Check sheet for the modelled part. Datum: model origin and axes. Units: mm. A direction names the side the tool comes from. Round coordinates to 2 decimals unless told otherwise and drop trailing zeros. Write each loop counter-clockwise with the first axis right and the second up, starting at its lowest first coordinate (ties: lowest second). Pieces come first, ordered by that corner, then holes.
Item 1: Tool access check on faces 1 (the flat face through (23.855, -8, 9)), 2 (the flat face through (10, 30.184, 9)), 3 (the flat face through (-5.901, 33, 7)). Record the directions out of +Z, -Z, +X, -X, +Y, -Y that give a thin tool (end or side, any length) a straight path to the whole face; none if there is none.
Item 2: Material ranges on line 1 (Y direction, x = -28, z = 3); line 2 (X direction, y = 34, z = 10); line 3 (X direction, y = -4, z = 10.75) (1 decimal), recorded low to high.
Item 3: Cross-section at A-A on y = -8. Enter the section's corners in (x, z) (3 decimals), plus the area to 3 significant figures.
Item 4: Cross-section at B-B on z = 1.5. Count the separate pieces of the cut face and the enclosed holes in it, plus the area to 3 significant figures.
Item 5: Release check for a two-part mould opening along X. For faces 4 (the flat face through (-21, 26, 2)), 5 (the flat face through (4.5, 1, 9)), 6 (the flat face through (33.5, 0, 2)), 7 (the cylindrical face through (-27.833, -20.894, 1.972)) record: +X half, -X half, draft (parallel to the pull), parting line (faces both ways), or undercut.
Item 6: Go/stop test with flat-tipped pins: pin 1 Ø3 at (x, z) = (30, 1.5) entering from +Y; pin 2 Ø1 at (y, z) = (9, 12) entering from -X; pin 3 Ø3 at (y, z) = (-9.5, 11) entering from +X (3 decimals); pin 4 Ø8 at (x, z) = (15.5, 10) entering from +Y. Record where each tip stops, or that it passes through.
from build123d import *

# Parameters (mm, degrees)
ESBO_O1_R                                       = 2.5
RESSALTO_EXTRUS_O1_DEPTH                        = 4
ESBO_O2_R                                       = 1.5
ESBO_O2_R_2                                     = 5
ESBO_O2_R_3                                     = 4
ESBO_O2_R_4                                     = 2
CORTE_EXTRUS_O1_DEPTH                           = 4
ESBO_O3_R                                       = 6.5
CUT_EXTRUDE1_DEPTH                              = 3
SKETCH1_R                                       = 2.5
BOSS_EXTRUDE1_DEPTH                             = 10
SKETCH2_R                                       = 1
CUT_EXTRUDE3_DEPTH                              = 58
CSK_FOR_M5_FLAT_HEAD_MACHINE_SCREW1_D           = 5.3
CSK_FOR_M5_FLAT_HEAD_MACHINE_SCREW1_CSINK_D     = 10.4
CSK_FOR_M5_FLAT_HEAD_MACHINE_SCREW1_CSINK_ANGLE = 90


with BuildPart() as part:
    # Esboço1 → Ressalto-extrusão1 (new body)
    with BuildSketch(Plane.XY):
        with BuildLine():
            Line((28.048564207, 26.000016667), (31.500000169, 26.000016667))
            ThreePointArc((31.500000169, 26.000016667), (32.914213731, 25.414230229), (33.500000169, 24.000016667))
            Line((33.500000169, 24.000016667), (33.500000169, -24.000016667))
            ThreePointArc((33.500000169, -24.000016667), (32.914213731, -25.414230229), (31.500000169, -26.000016667))
            Line((31.500000169, -26.000016667), (12.499999983, -26.000016667))
            ThreePointArc((12.499999983, -26.000016667), (11.410019713, -27.2255233), (10.134109695, -28.256046043))
            Line((10.134109695, -28.256046043), (-1.094109442, -28.256046043))
            ThreePointArc((-1.094109442, -28.256046043), (-2.37001946, -27.2255233), (-3.45999973, -26.000016667))
            Line((-3.45999973, -26.000016667), (-31.500000169, -26.000016667))
            ThreePointArc((-31.500000169, -26.000016667), (-32.914213731, -25.414230229), (-33.500000169, -24.000016667))
            Line((-33.500000169, -24.000016667), (-33.500000169, 24.000016667))
            ThreePointArc((-33.500000169, 24.000016667), (-32.914213731, 25.414230229), (-31.500000169, 26.000016667))
            Line((-31.500000169, 26.000016667), (-10.901, 26.000016667))
            ThreePointArc((-10.901, 26.000016667), (-7.365466094, 27.464482761), (-5.901, 31.000016667))
            Line((-5.901, 31.000016667), (-5.901, 35.181429851))
            ThreePointArc((-5.901, 35.181429851), (-4.143640687, 39.424070538), (0.099, 41.181429851))
            Line((0.099, 41.181429851), (13.048564207, 41.181429851))
            ThreePointArc((13.048564207, 41.181429851), (20.119632019, 38.252497663), (23.048564207, 31.181429851))
            Line((23.048564207, 31.181429851), (23.048564207, 31.000016667))
            ThreePointArc((23.048564207, 31.000016667), (24.513030301, 27.464482761), (28.048564207, 26.000016667))
        make_face()
        with Locations((0.099, 35.181429851)):
            Circle(ESBO_O1_R, mode=Mode.SUBTRACT)
        with Locations((17.855, -8)):
            Circle(ESBO_O1_R, mode=Mode.SUBTRACT)
    extrude(amount=RESSALTO_EXTRUS_O1_DEPTH)

    # Esboço2 → Corte-extrusão1 (cut)
    with BuildSketch(Plane(origin=(0, 0, 0), x_dir=(-1, 0, 0), z_dir=(0, 0, -1))):
        with Locations((-28.728359433, -4.920628891)):
            Circle(ESBO_O2_R)
        with Locations((16.423325421, 19.853563273)):
            Circle(ESBO_O2_R)
        with Locations((27.863004989, 3.986376213)):
            Circle(ESBO_O2_R)
        with Locations((26.447101695, -20.319132993)):
            Circle(ESBO_O2_R)
        with Locations((13.238926139, 3.805699557)):
            Circle(ESBO_O2_R_2)
        with Locations((-13.474000127, 23.181446518)):
            Circle(ESBO_O2_R_3)
        with Locations((-4.5, -20)):
            Circle(ESBO_O2_R_3)
        with Locations((-23, -20)):
            Circle(ESBO_O2_R_4)
        with Locations((5, -20)):
            Circle(ESBO_O2_R_4)
    extrude(amount=-CORTE_EXTRUS_O1_DEPTH, mode=Mode.SUBTRACT)

    # Esboço3 → Cut-Extrude1 (cut)
    with BuildSketch(Plane(origin=(0, 0, 0), x_dir=(-1, 0, 0), z_dir=(0, 0, -1))):
        with Locations((-13.474000127, 23.181446518)):
            Circle(ESBO_O3_R)
        with Locations((-4.5, -20)):
            Circle(ESBO_O3_R)
    extrude(amount=-CUT_EXTRUDE1_DEPTH, mode=Mode.SUBTRACT)

    # Sketch1 → Boss-Extrude1 (add)
    # profile 1 of 2: a face of its own
    with BuildSketch(Plane.XY.offset(4)):
        with BuildLine():
            Line((13.454, 16.18142986), (13.454, 0.181429851))
            Line((13.454, 0.181429851), (20.855, 0.181429851))
            ThreePointArc((20.855, 0.181429851), (22.976320344, -0.697249805), (23.855, -2.818570149))
            Line((23.855, -2.818570149), (23.855, -13.257131994))
            ThreePointArc((23.855, -13.257131994), (18.073755029, -10.98960381), (12.198145727, -12.999999991))
            Line((12.198145727, -12.999999991), (4.499999978, -12.999999991))
            Line((4.499999978, -12.999999991), (4.499999978, 15.330875804))
            ThreePointArc((4.499999978, 15.330875804), (5.148168847, 15.729461399), (5.76031088, 16.18142986))
            Line((5.76031088, 16.18142986), (13.454, 16.18142986))
        make_face()
        with Locations((17.855, -8)):
            Circle(SKETCH1_R, mode=Mode.SUBTRACT)
    # profile 2 of 2: a face of its own
    with BuildSketch(Plane.XY.offset(4)):
        with BuildLine():
            Line((13.453999976, 41.181429851), (0.099, 41.181429851))
            ThreePointArc((0.099, 41.181429851), (-4.143640687, 39.424070538), (-5.901, 35.181429851))
            Line((-5.901, 35.181429851), (-5.901, 31.000016667))
            ThreePointArc((-5.901, 31.000016667), (-5.944227937, 30.34395972), (-6.073164287, 29.699246768))
            ThreePointArc((-6.073164287, 29.699246768), (-0.248774232, 32.164172288), (5.757624044, 30.183627646))
            Line((5.757624044, 30.183627646), (13.453999976, 30.183627646))
            Line((13.453999976, 30.183627646), (13.453999976, 41.181429851))
        make_face()
        with Locations((0.099, 35.181429851)):
            Circle(SKETCH1_R, mode=Mode.SUBTRACT)
    extrude(amount=BOSS_EXTRUDE1_DEPTH)

    # Sketch2 → Cut-Extrude3 (cut)
    with BuildSketch(Plane(origin=(0, 41.181429851, 0), x_dir=(-1, 0, 0), z_dir=(0, 1, 0))):
        with Locations(Location((-8.993889952, 10.832314202, 0), (0, 0, 90))):
            Circle(SKETCH2_R)
    extrude(amount=-CUT_EXTRUDE3_DEPTH, mode=Mode.SUBTRACT)

    # CSK for M5 Flat Head Machine Screw1 (through all)
    with Locations(Plane(origin=(0, 0, 0), x_dir=(-1, 0, 0), z_dir=(0, 0, -1))):
        with Locations((-0.099, 35.181429851), (-17.855, -8)):
            CounterSinkHole(CSK_FOR_M5_FLAT_HEAD_MACHINE_SCREW1_D / 2, CSK_FOR_M5_FLAT_HEAD_MACHINE_SCREW1_CSINK_D / 2, counter_sink_angle=CSK_FOR_M5_FLAT_HEAD_MACHINE_SCREW1_CSINK_ANGLE)


solid = part.part
Response values:
1. face 1: +Z, +X, +Y, -Y
1. face 2: +Z, +X
1. face 3: +Z, -Z, -X, +Y
2. line 1: y = -26 to 2.49, 5.48 to 26
2. line 2: x = -5.9 to -2.27, 2.47 to 8.44, 9.55 to 13.45
2. line 3: x = 4.5 to 8, 10 to 23.9
3. outline: (-33.5, 0) - (12.655, 0) - (15.205, 2.55) - (15.205, 14) - (4.5, 14) - (4.5, 4) - (-33.5, 4) - close; (20.505, 2.55) - (23.055, 0) - (33.5, 0) - (33.5, 4) - (23.855, 4) - (23.855, 14) - (20.505, 14) - close; hole circle Ø2 at (8.994, 10.832)
3. area: 378 mm2
4. separate pieces: 1
4. enclosed holes: 11
4. area: 3,450 mm2
5. face 4: draft
5. face 5: -X half
5. face 6: +X half
5. face 7: undercut
6. pin 1: stops at y = 26
6. pin 2: stops at x = 4.5
6. pin 3: stops at x = 23.855
6. pin 4: stops at y = 41.18
